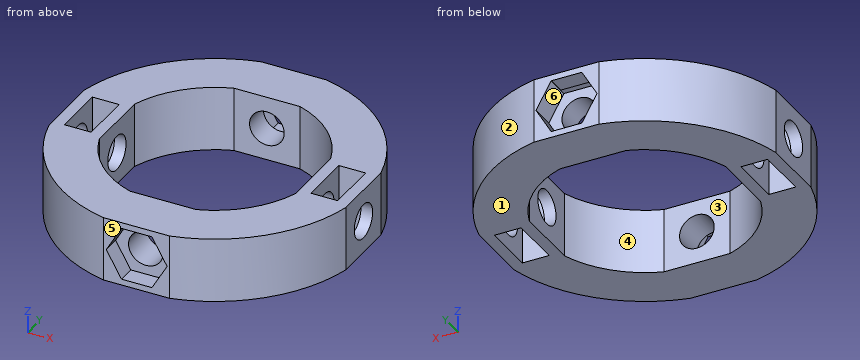
from build123d import *

# Parameters (mm, degrees)
PAD_DEPTH             = 10
SKETCH001_R           = 2.675
POCKET_DEPTH          = 7.776573
POCKET001_DEPTH       = 3.75
SKETCH003_W           = 4.15
SKETCH003_H           = 8.15
POCKET002_DEPTH       = 10
POLARPATTERN_COUNT    = 2
POLARPATTERN003_COUNT = 4
POCKET011_DEPTH       = 3.75


with BuildPart() as part:
    # Sketch → Pad (new body)
    with BuildSketch(Plane.XY):
        with BuildLine():
            Line((-22.935879, -5.118149), (-22.935879, 5.118149))
            ThreePointArc((-5, 22.961925), (-16.57418, 16.659729), (-22.935879, 5.118149))
            Line((-5, 22.961925), (5, 22.961925))
            ThreePointArc((22.935879, 5.118149), (16.57418, 16.659729), (5, 22.961925))
            Line((22.935879, 5.118149), (22.935879, -5.118149))
            ThreePointArc((5.118149, -22.935879), (16.617009, -16.617009), (22.935879, -5.118149))
            Line((-5.118149, -22.935879), (5.118149, -22.935879))
            ThreePointArc((-22.935879, -5.118149), (-16.617009, -16.617009), (-5.118149, -22.935879))
        make_face()
        with BuildLine():
            Line((-15.159306, 5.118149), (-15.159306, -5.118149))
            ThreePointArc((-15.159306, -5.118149), (-11.313708, -11.313708), (-5.118149, -15.159306))
            Line((-5.118149, -15.159306), (5.118149, -15.159306))
            ThreePointArc((5.118149, -15.159306), (11.313708, -11.313708), (15.159306, -5.118149))
            Line((15.159306, 5.118149), (15.159306, -5.118149))
            ThreePointArc((15.159306, 5.118149), (11.313708, 11.313708), (5.118149, 15.159306))
            Line((-5.118149, 15.159306), (5.118149, 15.159306))
            ThreePointArc((-5.118149, 15.159306), (-11.313708, 11.313708), (-15.159306, 5.118149))
        make_face(mode=Mode.SUBTRACT)
    extrude(amount=PAD_DEPTH)

    # Sketch001 (on Face7 of Pad) → Pocket (cut)
    with BuildSketch(Plane.XZ.offset(22.935879)):
        with Locations((0, 5)):
            Circle(SKETCH001_R)
    pocket = extrude(amount=-POCKET_DEPTH, mode=Mode.SUBTRACT)

    # Sketch002 → Pocket001 (cut)
    with BuildSketch(Plane.XZ.offset(23.958595)):
        Polygon((2.380832, 9.076277), (-2.324572, 9.076277), (-4.677275, 5.001277), (-2.324572, 0.926277), (2.380832, 0.926277), (4.733535, 5.001277), align=None)
    pocket001 = extrude(amount=-POCKET001_DEPTH, mode=Mode.SUBTRACT)

    # Sketch003 → Pocket002 (cut)
    with BuildSketch(Plane(origin=(0, 0, 0), x_dir=(1, 0, 0), z_dir=(0, 0, -1))):
        with Locations((-19.047593, 0)):
            Rectangle(SKETCH003_W, SKETCH003_H)
        with Locations((19.047593, 0)):
            Rectangle(SKETCH003_W, SKETCH003_H)
    extrude(amount=-POCKET002_DEPTH, mode=Mode.SUBTRACT)

    # PolarPattern: Pocket001 ×2 about axis
    polarpattern_axis = Axis((0, 0, 0), (0, 0, 1))
    for i in range(1, POLARPATTERN_COUNT):
        add(pocket001.rotate(polarpattern_axis, i * 360 / POLARPATTERN_COUNT), mode=Mode.SUBTRACT)

    # PolarPattern003: Pocket ×4 about axis
    polarpattern003_axis = Axis((0, 0, 0), (0, 0, 1))
    for i in range(1, POLARPATTERN003_COUNT):
        add(pocket.rotate(polarpattern003_axis, i * 360 / POLARPATTERN003_COUNT), mode=Mode.SUBTRACT)

    # Sketch014 (on Face8 of PolarPattern003) → Pocket011 (cut)
    with BuildSketch(Plane(origin=(0, 22.961925, 0), x_dir=(-1, 0, 0), z_dir=(0, 1, 0))):
        Polygon((4.705405, 5), (2.352702, 9.075), (-2.352702, 9.075), (-4.705405, 5), (-2.352702, 0.925), (2.352702, 0.925), align=None)
    extrude(amount=-POCKET011_DEPTH, mode=Mode.SUBTRACT)


solid = part.part
Source: CAD feature listing. Evaluate the final solid. Frame: model axes, mm. Face numbers are marked on the shaded views. A direction names the side the tool comes from. Give positions to 0.01 mm unless a question says otherwise; leave off trailing zeros. Write each loop counter-clockwise with the first axis right and the second up, starting at its lowest first coordinate (ties: lowest second). Pieces come first, ordered by that corner, then holes. Notation, with made-up numbers: (75.5, 38.25) -> (84.5, 38.25) arc R11 ccw to (84.5, 55.25) -> close; hole circle Ø6 at (74, -8). An arc over 180 degrees is marked (long way). Write item = value, one per line.
Q1. Cut plane D-D on y = -18.5. Return loops of the section in (x, z) (3 decimals).
Here are the results:
outline = (-14.491, 0) -> (14.491, 0) -> (14.491, 10) -> (-14.491, 10) -> close; hole circle Ø5.35 at (0, 5)
Q2. Cut plane A-A on x = 0. State how many separate pieces and enclosed holes the cut face has, then the cut area to 3 significant figures.
Here are the results:
separate_pieces = 4
enclosed_holes = 0
area = 54.3 mm²
Q3. Cut plane B-B on x = -8.5. Return loops of the section in (y, z), then the cut area to 3 significant figures.
Here are the results:
outline = (-21.91, 0) -> (-13.56, 0) -> (-13.56, 10) -> (-21.91, 10) -> close; (13.56, 0) -> (21.91, 0) -> (21.91, 10) -> (13.56, 10) -> close
area = 167 mm²
Q4. First-contact query: pin 1 (2 mm diameter, centred on x = -2, z = 7, fed in from +Y); pin 2 (6 mm diameter, centred on x = -16, z = 5.5, fed in from +Y); pin 3 (3 mm diameter, centred on y = -8, z = 7.5, fed in from +X); pin 4 (4.5 mm diameter, centred on x = 0, z = 5, fed in from +Y). Flat tips, straight axial feed; report the tip coordinate or a pass-through.
Here are the results:
pin_1 = 19.21
pin_2 = 19.58
pin_3 = 22.58
pin_4 = through
Q5. Cut plane C-C on y = 10.5. Return loops of the section in (x, z).
Here are the results:
outline = (-21.02, 0) -> (-12.07, 0) -> (-12.07, 10) -> (-21.02, 10) -> close; (12.07, 0) -> (21.02, 0) -> (21.02, 10) -> (12.07, 10) -> close
Q6. Line query: line 1 (X direction, y = 3, z = 5.5); line 2 (Z direction, x = 22.15, y = 0) (3 decimals); line 3 (Y direction, x = 4, z = 6). Output: solid intervals per line, ascending. Write a range as from..to.
Here are the results:
line_1 = -22.94..-21.12, -16.97..-15.16, 15.16..16.97, 21.12..22.94
line_2 = 0..2.325, 7.675..10
line_3 = -20.21..-15.16, 15.16..19.21
Q7. Reachability of the marked faces 4, 5 and 6 from +Z, -Z, +X, -X, +Y, -Y: full face, straight path, thin tool, end or side. Return the list, or none.
Here are the results:
face_4 = +Z, -Z
face_5 = +Z, -Z, +X, -X, -Y
face_6 = +Y
Q8. Mould query, pull axis Y, two halves, no side actions, for the marked faces 1, 2 and 3. Classes: +Y half, -Y half, draft (parallel to the pull), parting line (faces both ways), or undercut.
Here are the results:
face_1 = draft
face_2 = +Y half
face_3 = undercut
